```python
from build123d import *

# Parameters (mm, degrees)
BOSS_EXTRUDE1_DEPTH = 6.35
SKETCH2_R           = 5.08
CUT_EXTRUDE1_DEPTH  = 201.754423986
SKETCH3_R           = 2.159
CUT_EXTRUDE2_DEPTH  = 201.754423986
SKETCH6_R           = 2.159
CUT_EXTRUDE3_DEPTH  = 6.35


with BuildPart() as part:
    # Sketch1 → Boss-Extrude1 (new body)
    with BuildSketch(Plane(origin=(0, 0, 0), x_dir=(1, 0, 0), z_dir=(0, 1, 0))):
        with BuildLine():
            Line((-174.625, 12.7), (174.625, 12.7))
            ThreePointArc((174.625, 12.7), (200.025, 0), (174.625, -12.7))
            Line((174.625, -12.7), (-174.625, -12.7))
            ThreePointArc((-174.625, -12.7), (-200.025, 0), (-174.625, 12.7))
        make_face()
    extrude(amount=BOSS_EXTRUDE1_DEPTH)

    # Sketch2 → Cut-Extrude1 (cut, through all)
    with BuildSketch(Plane(origin=(0, 6.35, 0), x_dir=(1, 0, 0), z_dir=(0, 1, 0))):
        with Locations(Location((184.15, 0, 0), (0, 0, 270))):
            Circle(SKETCH2_R)
        with Locations(Location((-184.15, 0, 0), (0, 0, 90))):
            Circle(SKETCH2_R)
        with BuildLine():
            Line((173.691383345, 1.25), (175.608616655, 1.25))
            ThreePointArc((175.608616655, 1.25), (176.858616655, 0), (175.608616655, -1.25))
            Line((175.608616655, -1.25), (173.691383345, -1.25))
            ThreePointArc((173.691383345, -1.25), (172.441383345, 0), (173.691383345, 1.25))
        make_face()
        with BuildLine():
            Line((194.608616655, 1.25), (192.691383345, 1.25))
            ThreePointArc((192.691383345, 1.25), (191.441383345, 0), (192.691383345, -1.25))
            Line((192.691383345, -1.25), (194.608616655, -1.25))
            ThreePointArc((194.608616655, -1.25), (195.858616655, 0), (194.608616655, 1.25))
        make_face()
        with BuildLine():
            Line((185.4, 8.920928665), (185.4, 6.921035691))
            ThreePointArc((185.4, 6.921035691), (184.15, 5.671035691), (182.9, 6.921035691))
            Line((182.9, 6.921035691), (182.9, 8.920928665))
            ThreePointArc((182.9, 8.920928665), (184.15, 10.170928665), (185.4, 8.920928665))
        make_face()
        with BuildLine():
            Line((185.441381345, -9.078964309), (185.441381345, -7.078964309))
            ThreePointArc((185.441381345, -7.078964309), (184.191381345, -5.828964309), (182.941381345, -7.078964309))
            Line((182.941381345, -7.078964309), (182.941381345, -9.078964309))
            ThreePointArc((182.941381345, -9.078964309), (184.191381345, -10.328964309), (185.441381345, -9.078964309))
        make_face()
        with BuildLine():
            Line((-185.441381345, -9.078964309), (-185.441381345, -7.078964309))
            ThreePointArc((-185.441381345, -7.078964309), (-184.191381345, -5.828964309), (-182.941381345, -7.078964309))
            Line((-182.941381345, -7.078964309), (-182.941381345, -9.078964309))
            ThreePointArc((-182.941381345, -9.078964309), (-184.191381345, -10.328964309), (-185.441381345, -9.078964309))
        make_face()
        with BuildLine():
            Line((-185.4, 8.920928665), (-185.4, 6.921035691))
            ThreePointArc((-185.4, 6.921035691), (-184.15, 5.671035691), (-182.9, 6.921035691))
            Line((-182.9, 6.921035691), (-182.9, 8.920928665))
            ThreePointArc((-182.9, 8.920928665), (-184.15, 10.170928665), (-185.4, 8.920928665))
        make_face()
        with BuildLine():
            Line((-194.608616655, 1.25), (-192.691383345, 1.25))
            ThreePointArc((-192.691383345, 1.25), (-191.441383345, 0), (-192.691383345, -1.25))
            Line((-192.691383345, -1.25), (-194.608616655, -1.25))
            ThreePointArc((-194.608616655, -1.25), (-195.858616655, 0), (-194.608616655, 1.25))
        make_face()
        with BuildLine():
            Line((-173.691383345, 1.25), (-175.608616655, 1.25))
            ThreePointArc((-175.608616655, 1.25), (-176.858616655, 0), (-175.608616655, -1.25))
            Line((-175.608616655, -1.25), (-173.691383345, -1.25))
            ThreePointArc((-173.691383345, -1.25), (-172.441383345, 0), (-173.691383345, 1.25))
        make_face()
    extrude(amount=-CUT_EXTRUDE1_DEPTH, mode=Mode.SUBTRACT)

    # Sketch3 → Cut-Extrude2 (cut, through all)
    with BuildSketch(Plane(origin=(0, 6.35, 0), x_dir=(1, 0, 0), z_dir=(0, 1, 0))):
        with Locations(Location((0, 0, 0), (0, 0, 270))):
            Circle(SKETCH3_R)
        with Locations(Location((38.1, 0, 0), (0, 0, 270))):
            Circle(SKETCH3_R)
        with Locations(Location((-38.1, 0, 0), (0, 0, 270))):
            Circle(SKETCH3_R)
    extrude(amount=-CUT_EXTRUDE2_DEPTH, mode=Mode.SUBTRACT)

    # Sketch6 → Cut-Extrude3 (cut)
    with BuildSketch(Plane(origin=(0, 0, 0), x_dir=(-1, 0, 0), z_dir=(0, -1, 0))):
        with Locations(Location((54.61, 0, 0), (0, 0, 90))):
            Circle(SKETCH6_R)
        with Locations(Location((-54.61, 0, 0), (0, 0, 90))):
            Circle(SKETCH6_R)
    extrude(amount=-CUT_EXTRUDE3_DEPTH, mode=Mode.SUBTRACT)


solid = part.part
```
Input: part model. Units: mm. Frame: model coordinates. A direction names the side the tool comes from. Give positions to 0.01 mm unless a question says otherwise; leave off trailing zeros. Loops run counter-clockwise (first coordinate to the right, second up) from the corner with the lowest first, then second, coordinate; pieces in that order, holes last.
1) Mould query, pull axis X, two halves, no side actions, for faces 4 (the cylindrical face through (-179.19, 3.22, 1.1)), 5 (the flat face through (3, 0, 0)). Classes: released by +X, released by -X, zero draft, split by the parting line, or undercut.
A:
face 4: undercut
face 5: zero draft
2) Reachability of faces 1 (the cylindrical face through (179.19, 3.22, -1.1)), 2 (the flat face through (2, 3, 12.7)), 3 (the flat face through (-2, 3, -12.7)) from +Z, -Z, +X, -X, +Y, -Y: full face, straight path, thin tool, end or side. Return the list, or none.
A:
face 1: +Y, -Y
face 2: +Z, +Y, -Y
face 3: -Z, +Y, -Y
3) Section query B-B on x = 134.5. Return the cut outline in (y, z), and give its area (3 significant figures).
A:
outline: (0, -12.7) - (6.35, -12.7) - (6.35, 12.7) - (0, 12.7) - close
area: 161 mm2
4) Contact query for flat-ended pins moving along their axis: pin 1 (2 mm diameter, centred on x = -194, y = 3.5, fed in from +Z); pin 2 (2 mm diameter, centred on x = 194, y = 3, fed in from -Z); pin 3 (1.5 mm diameter, centred on x = 193.5, y = 2.5, fed in from +Z). Output: stop coordinate, or through.
A:
pin 1: stops at z = 13.18
pin 2: stops at z = -13.18
pin 3: stops at z = 13.34
5) Line query: L1, parallel to X at y = 1.75, z = -6.5; L2, parallel to X at y = 5, z = 3.5; L3, parallel to Z at x = 31.5, y = 5. Output: solid intervals per line, ascending.
A:
L1: x = -198.63 to -185.33, -182.97 to 182.97, 185.33 to 198.63
L2: x = -199.63 to -187.83, -180.47 to 180.47, 187.83 to 199.63
L3: z = -12.7 to 12.7
6) Section query A-A on y = 4.5. Count the separate pieces of the cut face and the enclosed holes in it, and give its area (3 significant figures).
A:
separate pieces: 1
enclosed holes: 15
area: 9,920 mm2
